from build123d import *

# Parameters (mm, degrees)
EXTRUDE_THIN1_DEPTH = 762
FILLET1_R           = 1.27


with BuildPart() as part:
    # Sketch1 → Extrude-Thin1 (new body)
    with BuildSketch(Plane.XY):
        with BuildLine():
            Line((0, 0), (0, -3.175))
            Line((0, -3.175), (-21.43125, -3.175))
            ThreePointArc((-21.43125, -3.175), (-25.921378, -5.034872), (-27.78125, -9.525))
            Line((-27.78125, -9.525), (-34.528125, -9.525))
            Line((-34.528125, -9.525), (-34.528125, 15.875))
            Line((-34.528125, 15.875), (-38.89375, 15.875))
            Line((-38.89375, 15.875), (-38.89375, 22.225))
            ThreePointArc((-38.89375, 22.225), (-44.544809, 24.082461), (-47.991853, 28.9304))
            Line((-47.991853, 28.9304), (-52.814397, 44.491475))
            ThreePointArc((-52.814397, 44.491475), (-56.261441, 49.339414), (-61.9125, 51.196875))
            Line((-61.9125, 51.196875), (-61.9125, 66.675))
            Line((-61.9125, 66.675), (-55.00013, 66.675))
            ThreePointArc((-55.00013, 66.675), (-52.755066, 66.264881), (-50.8, 65.0875))
            Line((-50.8, 65.0875), (-51.640026, 64.135))
            ThreePointArc((-51.640026, 64.135), (-53.204079, 65.076905), (-55.00013, 65.405))
            Line((-55.00013, 65.405), (-60.6425, 65.405))
            Line((-60.6425, 65.405), (-60.6425, 52.391909))
            ThreePointArc((-60.6425, 52.391909), (-55.007036, 49.96926), (-51.601316, 44.867421))
            Line((-51.601316, 44.867421), (-46.778773, 29.306347))
            ThreePointArc((-46.778773, 29.306347), (-43.264039, 24.746743), (-37.62375, 23.593277))
            Line((-37.62375, 23.593277), (-37.62375, 17.145))
            Line((-37.62375, 17.145), (-33.258125, 17.145))
            Line((-33.258125, 17.145), (-33.258125, -8.255))
            Line((-33.258125, -8.255), (-28.944671, -8.255))
            ThreePointArc((-28.944671, -8.255), (-26.349939, -3.705129), (-21.43125, -1.905))
            Line((-21.43125, -1.905), (-1.27, -1.905))
            Line((-1.27, -1.905), (-1.27, 0))
            Line((-1.27, 0), (0, 0))
        make_face()
    extrude(amount=-EXTRUDE_THIN1_DEPTH)

    # Fillet1
    fillet1_edges = [part.edges().sort_by_distance(p)[0] for p in [
        (-37.62375, 23.593277, -381),
        (-33.258125, 17.145, -381),
        (0, -3.175, -381),
        (-27.78125, -9.525, -381),
        (-34.528125, -9.525, -381),
        (-38.89375, 15.875, -381),
        (-61.9125, 51.196875, -381),
        (-61.9125, 66.675, -381),
    ]]
    fillet(fillet1_edges, radius=FILLET1_R)


solid = part.part
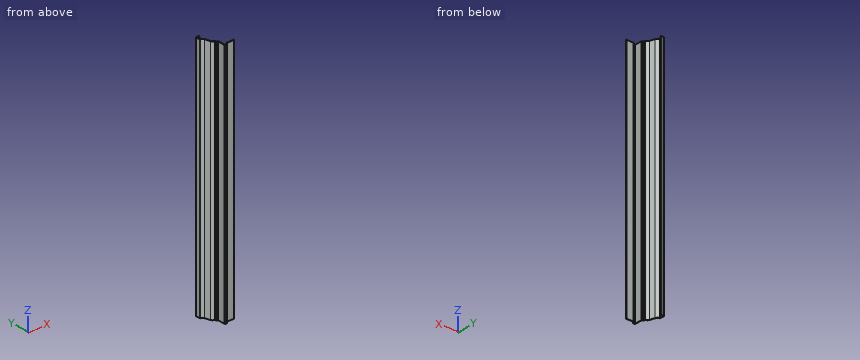
Input: part model. Units: mm. Frame: model coordinates. Coordinates: 2 decimals unless noted, no trailing zeros. Write each loop counter-clockwise with the first axis right and the second up, starting at its lowest first coordinate (ties: lowest second). Pieces come first, ordered by that corner, then holes. Notation, with made-up numbers: M 54.25,50 L 85.25,50 A26 ccw 85.25,76 Z; hole C 83.5,65.5 d2. An arc over 180 degrees is marked long. Answer as a JSON object with one key per item and string values. Group by question number.
(1) Section B-B on y = 38. Output: boundary loops of the cut face in (x, z).
(2) Contact query for flat-ended pins moving along their axis: P1, Ø12, axis at x = -13, z = -148, coming from the +Y side (3 decimals); P2, Ø1.5, axis at x = -36.5, z = -505.5, coming from the +Y side (3 decimals); P3, Ø6, axis at x = -13.5, z = -213, coming from the -Y side (3 decimals); P4, Ø19.5, axis at y = 8, z = -248, coming from the +X side. Output: stop coordinate, or through.
(3) Ray query, line 1 along X through (y, z) = (59.5, -583.5); line 2 along Y through (x, z) = (-16, -404) (3 decimals); line 3 along Y through (x, z) = (-32, -161) (3 decimals). Return the intervals inside material, ascending. Write a range as [from, to].
(4) Section A-A on x = -13. Output: boundary loops of the cut face in (y, z) (3 decimals).
Result set:
{
 "1": {"outline": "M -50.8,-762 L -49.47,-762 L -49.47,0 L -50.8,0 Z"},
 "2": {"P1": "stops at y = -1.905", "P2": "stops at y = 17.145", "P3": "stops at y = -3.175", "P4": "stops at x = 0"},
 "3": {"line 1": "x = [-61.91, -60.64]", "line 2": "y = [-3.175, -1.905]", "line 3": "y = [-9.525, -8.255]"},
 "4": {"outline": "M -3.175,-762 L -1.905,-762 L -1.905,0 L -3.175,0 Z"}
}
